Answer from the drawing. Dimensions are ordinates in mm from the lowest x, y and z of the part. Coordinates: 2 decimals unless noted, no trailing zeros. Order: outer loops, then holes, each group sorted by start corner. A loop starts at its lowest first (then second) coordinate and runs counter-clockwise, first axis right, second up. Notation, with made-up numbers: M 6.5,-23 L 36.5,-23 A16 ccw 36.5,5 Z; hole C -40,-21 d1. An arc over 180 degrees is marked long. One line per question, with ' | ' between items. Start each with the question number.
1) Find section C-C, the plane y = 14. Write down the section's boundary in (x, z).
2) Consider probe 1 along Y at (x, z) = (145.5, 9.75); probe 2 along Y at (x, z) = (9, 14.25) (1 decimal); probe 3 along Y at (x, z) = (89, 2.8). Determine where each line is inside the solid, lowest interval first.
3) Find section A-A, the plane x = 80. Write down the section's boundary in (y, z).
4) Find section D-D, the plane z = 8.75. Write down the section's boundary in (x, y).
5) The mould has two halves that part along X. Classify the marked faces 1, 2 and 3: +X half, -X half, draft (parallel to the pull), parting line (faces both ways), or undercut.
6) Find section B-B, the plane y = 53. Write down the section's boundary in (x, z), plus the area to 3 significant figures.
7) Given P1, Ø6.5, axis at x = 70.5, y = 158, coming from the +Z side; P2, Ø16.5, axis at x = 120.5, y = 28.5, coming from the +Z side; P3, Ø2, axis at y = 55.5, z = 2, coming from the -X side; P4, Ø3, axis at x = 7, z = 8.5, coming from the +Y side (1 decimal), each flat-ended and moving along its own axis, determine where each tip first touches the part or whether it passes through.
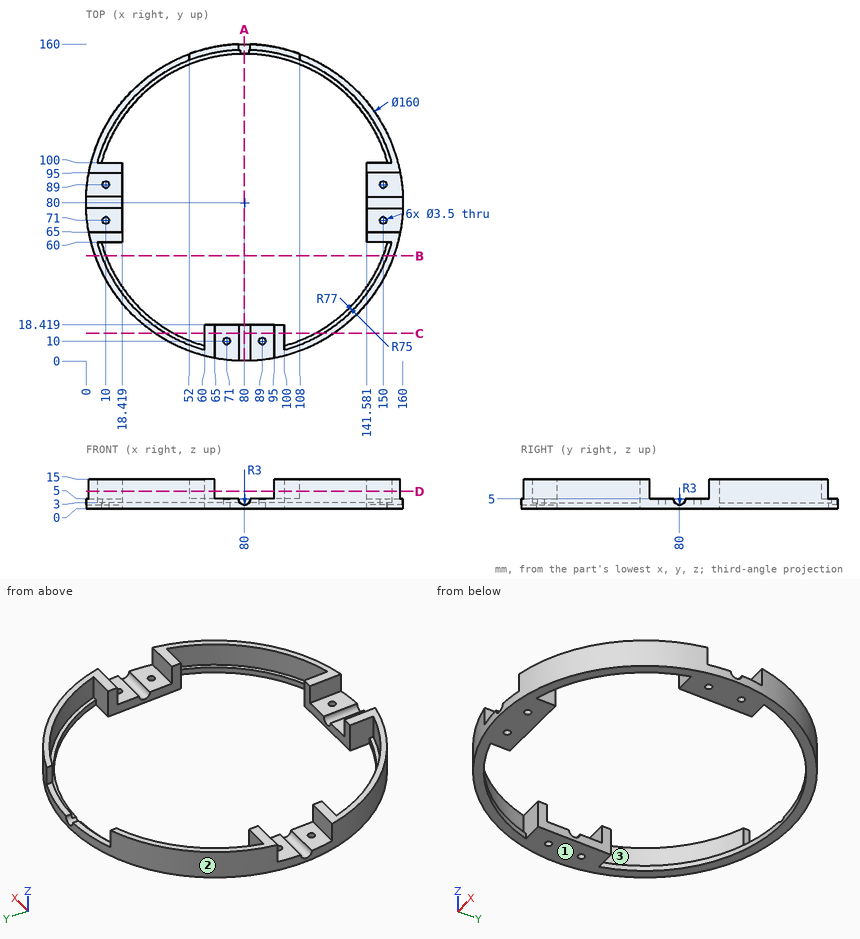
Report:
1) outline: M 34.79,0 L 44.38,0 L 44.38,3 L 40.34,3 L 40.34,15 L 34.79,15 Z; M 60,0 L 100,0 L 100,15 L 95,15 L 95,5 L 83,5 A3 cw 77,5 L 65,5 L 65,15 L 60,15 Z; M 115.62,0 L 125.21,0 L 125.21,15 L 119.66,15 L 119.66,3 L 115.62,3 Z
2) probe 1: y = 34.07 to 39.52, 60 to 65, 95 to 100, 120.48 to 125.93 | probe 2: y = 43.1 to 50.2, 60 to 65, 95 to 100, 109.8 to 116.9 | probe 3: y = 0.51 to 8.25, 11.75 to 18.42, 154.46 to 159.49
3) outline: M 0,0 L 18.42,0 L 18.42,2 L 0,2 Z; M 155,0 L 160,0 L 160,2 L 155,2 Z
4) outline: M 1.42,65 A80 ccw 65,1.42 L 65,18.42 L 60,18.42 L 60,5.64 A77 cw 5.64,60 L 18.42,60 L 18.42,65 Z; M 1.42,95 L 18.42,95 L 18.42,100 L 5.64,100 A77 cw 52,151.73 L 52,154.94 A80 ccw Z; M 95,1.42 A80 ccw 158.58,65 L 141.58,65 L 141.58,60 L 154.36,60 A77 cw 100,5.64 L 100,18.42 L 95,18.42 Z; M 108,151.73 A77 cw 154.36,100 L 141.58,100 L 141.58,95 L 158.58,95 A80 ccw 108,154.94 Z
5) face 1: draft | face 2: parting line | face 3: undercut
6) outline: M 4.69,0 L 10.03,0 L 10.03,3 L 7.89,3 L 7.89,15 L 4.69,15 Z; M 149.97,0 L 155.31,0 L 155.31,15 L 152.11,15 L 152.11,3 L 149.97,3 Z | area: 109 mm^2
7) P1: stops at z = 5 | P2: passes through | P3: stops at x = 3.53 | P4: stops at y = 115.9
